Verification items for the finished model (mm, model axes). A direction names the side the tool comes from. Give positions to 0.01 mm unless a question says otherwise; leave off trailing zeros. Write each loop counter-clockwise with the first axis right and the second up, starting at its lowest first coordinate (ties: lowest second). Pieces come first, ordered by that corner, then holes.
from build123d import *

# Parameters (mm, degrees)
BOSS_EXTRUDE1_DEPTH = 17
CUT_EXTRUDE1_REACH  = 9.2


with BuildPart() as part:
    # Sketch2 → Boss-Extrude1 (new body)
    with BuildSketch(Plane(origin=(0, 0, 0), x_dir=(1, 0, 0), z_dir=(0, 1, 0))):
        with BuildLine():
            Line((0, 0), (25, 0))
            ThreePointArc((25, 0), (12.5, -7.2), (0, 0))
        make_face()
    extrude(amount=BOSS_EXTRUDE1_DEPTH)

    # Sketch3 → Cut-Extrude1 (cut, up to next)
    with BuildSketch(Plane(origin=(0, 0, 0), x_dir=(-1, 0, 0), z_dir=(0, 0, -1)), mode=Mode.PRIVATE) as cut_extrude1_sk1:
        with BuildLine():
            Line((-15.75, 0), (-15.75, 6.75))
            ThreePointArc((-15.75, 6.75), (-12.5, 10), (-9.25, 6.75))
            Line((-9.25, 6.75), (-9.25, 0))
            Line((-9.25, 0), (-15.75, 0))
        make_face()
    cut_extrude1_tool1 = extrude(cut_extrude1_sk1.sketch, amount=-CUT_EXTRUDE1_REACH, mode=Mode.PRIVATE) & part.part
    add(cut_extrude1_tool1.solids().sort_by_distance((12.5, 4.679554, 0))[0], mode=Mode.SUBTRACT)


solid = part.part
Item 1: Sectioned sample at B-B on x = 12.5. Record the cut outline in (y, z), then the cut area to 3 significant figures.
Answer key:
outline: (10, 0) - (17, 0) - (17, 7.2) - (10, 7.2) - close
area: 50.4 mm2
Item 2: Sectioned sample at C-C on y = 15. Record the cut outline in (x, z).
Answer key:
outline: (0, 0) - (25, 0) arc R14.45 ccw to start
Item 3: Sectioned sample at A-A on z = 1.5. Record the cut outline in (x, y).
Answer key:
outline: (1, 0) - (9.25, 0) - (9.25, 6.75) arc R3.25 cw to (15.75, 6.75) - (15.75, 0) - (24, 0) - (24, 17) - (1, 17) - close
Item 4: Sectioned sample at D-D on z = 4.75. Record the cut outline in (x, y), then the cut area to 3 significant figures.
Answer key:
outline: (4.45, 0) - (9.25, 0) - (9.25, 6.75) arc R3.25 cw to (15.75, 6.75) - (15.75, 0) - (20.55, 0) - (20.55, 17) - (4.45, 17) - close
area: 213 mm2
Item 5: Release check for a two-part mould opening along X. For faces 1 (the face through (9.25, 3, 3)), 2 (the face through (12.7, 10.3, 7.2)), 3 (the face through (13, 17, 3)) record: released by +X, released by -X, zero draft, split by the parting line, or undercut.
Answer key:
face 1: undercut
face 2: split by the parting line
face 3: zero draft
Item 6: Depth check by flat-ended pin: pin 1 (2 mm diameter, centred on y = 4.5, z = 5, fed in from -X); pin 2 (1.5 mm diameter, centred on y = 14, z = 5.5, fed in from +X); pin 3 (2 mm diameter, centred on y = 3, z = 4.5, fed in from +X). Enter the tip coordinate at first touch or a pass-through.
Answer key:
pin 1: stops at x = 3.43
pin 2: stops at x = 20.55
pin 3: stops at x = 22.16
Item 7: Set-up check for faces 4 (the face through (15.75, 3, 3)), 5 (the face through (12.3, 10.3, 0)): record each of +Z, -Z, +X, -X, +Y, -Y from which the full face is reachable in a straight line by a thin tool's end or side.
Answer key:
face 4: +Z, -Z, -Y
face 5: -Z, +X, -X, +Y, -Y
Item 8: Scan lines: line 1 along X through (y, z) = (6.5, 5.25); line 2 along X through (y, z) = (5.25, 2); line 3 along Z through (x, y) = (22.5, 8.5). Record each from-to range of solid material in increasing order.
Answer key:
line 1: x = 5.25 to 9.25, 15.75 to 19.75
line 2: x = 1.4 to 9.25, 15.75 to 23.6
line 3: z = 0 to 3.18
